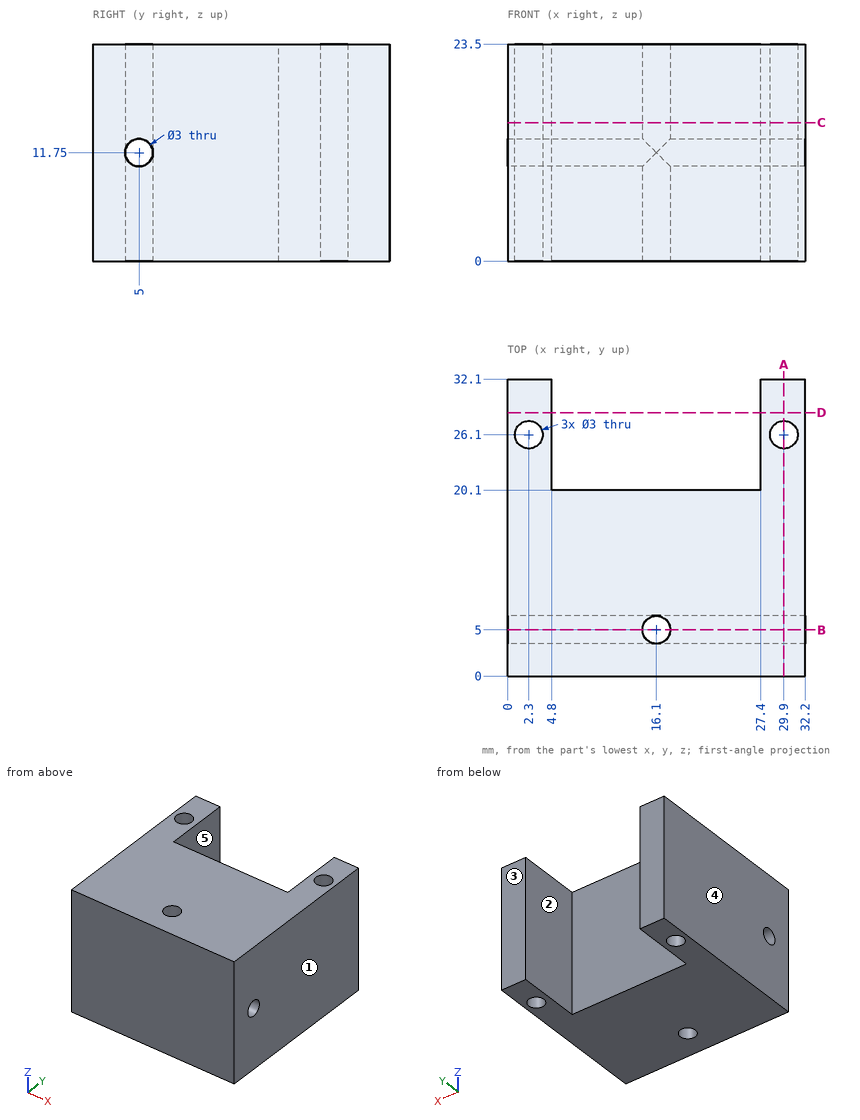
The figure shows three views and two pictorial views of one solid part (mm, origin at its lowest corner). Answer the questions. A direction names the side the tool comes from. Round coordinates to 2 decimals unless told otherwise and drop trailing zeros. Write each loop counter-clockwise with the first axis right and the second up, starting at its lowest first coordinate (ties: lowest second). Pieces come first, ordered by that corner, then holes. Notation, with made-up numbers: M 12.5,-6.75 L 48.5,-6.75 A20 ccw 48.5,22.25 Z; hole C -24,69.25 d6. An arc over 180 degrees is marked long. Use a Markdown table: item, result.
1) Flat-ended cylindrical pins translate along their axes: pin 1 (6 mm diameter, centred on x = 21.5, y = 26, fed in from +Z); pin 2 (3 mm diameter, centred on x = 22, z = 11, fed in from +Y). Find the tip coordinate at first contact, or state that the pin passes through.
Taken from the geometry:
| item | result |
|---|---|
| pin 1 | passes through |
| pin 2 | stops at y = 20.1 |
2) The part is cut by section C-C on z = 15. Give the vertices of the cut face in (x, y), plus the area to 3 significant figures.
Taken from the geometry:
| item | result |
|---|---|
| outline | M 0,0 L 32.2,0 L 32.2,32.1 L 27.4,32.1 L 27.4,20.1 L 4.8,20.1 L 4.8,32.1 L 0,32.1 Z; hole C 2.3,26.1 d3; hole C 16.1,5 d3; hole C 29.9,26.1 d3 |
| area | 741 mm2 |
3) Determine the mould class of the marked faces 3, 4 and 5 for opening direction X: pulls with the +X half, pulls with the -X half, needs draft (parallel to the pull), parting line crosses it, or undercut.
Taken from the geometry:
| item | result |
|---|---|
| face 3 | needs draft |
| face 4 | pulls with the -X half |
| face 5 | undercut |
4) Which of the six approach directions +Z, -Z, +X, -X, +Y, -Y give full straight-line access (tool end or side, diameter ignored) to the marked faces 1 and 2?
Taken from the geometry:
| item | result |
|---|---|
| face 1 | +Z, -Z, +X, +Y, -Y |
| face 2 | +Z, -Z, +Y |
5) Consider line 1 (X direction, y = 26, z = 8); line 2 (X direction, y = 5, z = 8.5); line 3 (Y direction, x = 16.1, z = 19). Determine where each line is inside the solid, lowest interval first. Write a range as [from, to].
Taken from the geometry:
| item | result |
|---|---|
| line 1 | x = [0, 0.8], [3.8, 4.8], [27.4, 28.4], [31.4, 32.2] |
| line 2 | x = [0, 14.6], [17.6, 32.2] |
| line 3 | y = [0, 3.5], [6.5, 20.1] |
6) The part is cut by section D-D on y = 28.5. Give the vertices of the cut face in (x, z).
Taken from the geometry:
| item | result |
|---|---|
| outline | M 0,0 L 4.8,0 L 4.8,23.5 L 0,23.5 Z; M 27.4,0 L 32.2,0 L 32.2,23.5 L 27.4,23.5 Z |
7) The part is cut by section B-B on y = 5. Give the vertices of the cut face in (x, z), plus the area to 3 significant figures.
Taken from the geometry:
| item | result |
|---|---|
| outline | M 0,0 L 14.6,0 L 14.6,10.25 L 0,10.25 Z; M 0,13.25 L 14.6,13.25 L 14.6,23.5 L 0,23.5 Z; M 17.6,0 L 32.2,0 L 32.2,10.25 L 17.6,10.25 Z; M 17.6,13.25 L 32.2,13.25 L 32.2,23.5 L 17.6,23.5 Z |
| area | 599 mm2 |
8) The part is cut by section A-A on x = 29.9. Give the vertices of the cut face in (y, z), plus the area to 3 significant figures.
Taken from the geometry:
| item | result |
|---|---|
| outline | M 0,0 L 24.6,0 L 24.6,23.5 L 0,23.5 Z; M 27.6,0 L 32.1,0 L 32.1,23.5 L 27.6,23.5 Z; hole C 5,11.75 d3 |
| area | 677 mm2 |
